Part model, mm, in its own coordinate system. A direction names the side the tool comes from. Give positions to 0.01 mm unless a question says otherwise; leave off trailing zeros. Order: outer loops, then holes, each group sorted by start corner. A loop starts at its lowest first (then second) coordinate and runs counter-clockwise, first axis right, second up.
1. Probe line 1 (Y direction, x = 15, z = 4); line 2 (X direction, y = -1.75, z = 5); line 3 (Z direction, x = 0, y = -2.5). List the from-to ranges inside material, lowest first.
2. Drop flat-ended pins along their axis: pin 1 Ø4 at (y, z) = (-3, -6) entering from +X; pin 2 Ø1 at (y, z) = (0, -10.5) entering from +X; pin 3 Ø1.6 at (x, y) = (-5.5, -1) entering from +Z. Give the stop position or say it passes through.
3. Slice it at D-D on z = 3.5. List the corners of the cut face in (x, y).
4. Slice it at B-B on z = 0. List the corners of the cut face in (x, y), and give its area (3 significant figures).
5. Slice it at C-C on y = 0.75. List the corners of the cut face in (x, z), and give its area (3 significant figures).
6. Which spindle directions (+Z, -Z, +X, -X, +Y, -Y) get a long thin tool onto all of the face, cutting with end or side? Do faces 5 (the flat face through (4, -4.5, -4)), 6 (the flat face through (-3, -1, 8)). Say none if no direction does.
7. Slice it at A-A on x = 0. List the corners of the cut face in (y, z).
8. Mould opens along Y. For faces 1 (the cylindrical face through (-14.985, -0.986, 0.66)), 2 (the flat face through (-4, 2.5, -4)), 3 (the cylindrical face through (0.867, -0.951, -3.905)), 4 (the flat face through (6, -2, 7)) say: +Y half, -Y half, draft (parallel to the pull), parting line (faces both ways), or undercut.
from build123d import *

# Parameters (mm, degrees)
F0_R     = 15
F1_DEPTH = 2
F2_R     = 17.5
F3_DEPTH = 2.5
F4_R     = 17.5
F5_DEPTH = 2.5
F7_D     = 8


with BuildPart() as f1:
    # F0 (on Front) → F1 (new body)
    with BuildSketch(Plane.XZ):
        Circle(F0_R)
        with BuildLine():
            Line((-3, -3), (-3, -12.134661))
            ThreePointArc((-3, -12.134661), (-8.838835, -8.838835), (-12.134661, -3))
            Line((-12.134661, -3), (-3, -3))
        make_face(mode=Mode.SUBTRACT)
        with BuildLine():
            Line((3, -12.134661), (3, -3))
            Line((3, -3), (12.134661, -3))
            ThreePointArc((12.134661, -3), (8.838835, -8.838835), (3, -12.134661))
        make_face(mode=Mode.SUBTRACT)
        with BuildLine():
            ThreePointArc((-12.134661, 3), (-8.838835, 8.838835), (-3, 12.134661))
            Line((-3, 12.134661), (-3, 3))
            Line((-3, 3), (-12.134661, 3))
        make_face(mode=Mode.SUBTRACT)
        with BuildLine():
            Line((12.134661, 3), (3, 3))
            Line((3, 3), (3, 12.134661))
            ThreePointArc((3, 12.134661), (8.838835, 8.838835), (12.134661, 3))
        make_face(mode=Mode.SUBTRACT)
    extrude(amount=F1_DEPTH)

    # F2 (on face) → F3 (join)
    with BuildSketch(Plane(origin=(0, 0, 0), x_dir=(-1, 0, 0), z_dir=(0, 1, 0))):
        Circle(F2_R)
    extrude(amount=F3_DEPTH)

    # F4 (on face) → F5 (join)
    with BuildSketch(Plane.XZ.offset(2)):
        Circle(F4_R)
    extrude(amount=F5_DEPTH)

    # F7 (through all)
    with Locations(Plane.XZ.offset(4.5)):
        with Locations((0, 0)):
            Hole(F7_D / 2)


solid = f1.part
Data:
1. line 1: y = -4.5 to -2, 0 to 2.5
1. line 2: x = -14.14 to -11.46, -3 to 3, 11.46 to 14.14
1. line 3: z = -17.5 to -4, 4 to 17.5
2. pin 1: stops at x = 17.04
2. pin 2: stops at x = 14.36
2. pin 3: stops at z = 14.24
3. outline: (-17.15, -4.5) - (-1.94, -4.5) - (-1.94, 2.5) - (-17.15, 2.5) - (-17.15, 0) - (-14.59, 0) - (-14.59, -2) - (-17.15, -2) - close; (1.94, -4.5) - (17.15, -4.5) - (17.15, -2) - (14.59, -2) - (14.59, 0) - (17.15, 0) - (17.15, 2.5) - (1.94, 2.5) - close; hole (-12, -2) - (-3, -2) - (-3, 0) - (-12, 0) - close; hole (3, -2) - (12, -2) - (12, 0) - (3, 0) - close
4. outline: (-17.5, -4.5) - (-4, -4.5) - (-4, 2.5) - (-17.5, 2.5) - (-17.5, 0) - (-15, 0) - (-15, -2) - (-17.5, -2) - close; (4, -4.5) - (17.5, -4.5) - (17.5, -2) - (15, -2) - (15, 0) - (17.5, 0) - (17.5, 2.5) - (4, 2.5) - close
4. area: 179 mm2
5. outline: circle Ø35 at (0, 0); hole circle Ø8 at (0, 0)
5. area: 912 mm2
6. face 5: +Z, -Z, +X, -X, -Y
6. face 6: none
7. outline: (-4.5, -17.5) - (-2, -17.5) - (-2, -15) - (0, -15) - (0, -17.5) - (2.5, -17.5) - (2.5, -4) - (-4.5, -4) - close; (-4.5, 4) - (2.5, 4) - (2.5, 17.5) - (0, 17.5) - (0, 15) - (-2, 15) - (-2, 17.5) - (-4.5, 17.5) - close
8. face 1: undercut
8. face 2: +Y half
8. face 3: draft
8. face 4: undercut
